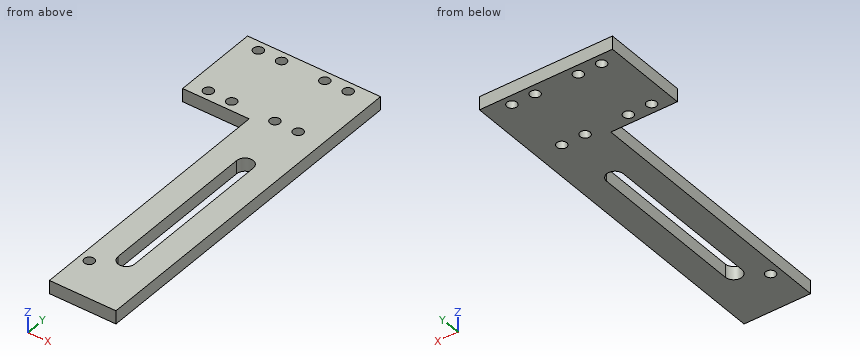
Autodesk Inventor part; units mm, degrees
ref_plane "YZ Plane" through (0, 0, 0) normal (1, 0, 0) x (0, 1, 0)
ref_plane "XZ Plane" through (0, 0, 0) normal (0, 1, 0) x (-1, 0, 0)
ref_plane "XY Plane" through (0, 0, 0) normal (0, 0, 1) x (1, 0, 0)
sketch "Skizze1" plane through (0, 0, 0) normal (0, 0, 1) x (1, 0, 0)
  line L0 (0, 0) -> (0, 80)
  line L1 (0, 80) -> (-20, 80)
  line L2 (-20, 80) -> (-20, 106)
  line L3 (-20, 106) -> (20, 106)
  line L4 (20, 106) -> (20, 0)
  line L5 (20, 0) -> (0, 0)
  arc A0 (7.5, 17.5) -> (12.5, 17.5) centre (10, 17.5) ccw
  arc A1 (12.5, 65) -> (7.5, 65) centre (10, 65) ccw
  line L6 (7.5, 65) -> (7.5, 17.5)
  line L7 (12.5, 65) -> (12.5, 17.5)
  dimension "d0" = 26
  dimension "d1" = 80
  dimension "d2" = 40
  dimension "d3" = 20
  dimension "d5" = 5
  dimension "d6" = 15
  dimension "d7" = 10
  dimension "d8" = 10
  dimension "d9" = 65
  dimension "d12" = 2.5
extrude "Extrusion1" add sketch "Skizze1" along normal blind 4
hole "Bohrung1" at (-14.5, 83, 4) direction (0, 0, -1) diameter 3 depth 8 tip angle 118
hole "Bohrung2" at (-7.5, 83, 4) direction (0, 0, -1) diameter 3 depth 8 tip angle 118
hole "Bohrung3" at (5.5, 83, 4) direction (0, 0, -1) diameter 3 depth 8 tip angle 118
hole "Bohrung4" at (12.5, 83, 4) direction (0, 0, -1) diameter 3 depth 8 tip angle 118
hole "Bohrung5" at (-14.5, 103, 4) direction (0, 0, -1) diameter 3 depth 8 tip angle 118
hole "Bohrung6" at (-7.5, 103, 4) direction (0, 0, -1) diameter 3 depth 8 tip angle 118
hole "Bohrung7" at (5.5, 103, 4) direction (0, 0, -1) diameter 3 depth 8 tip angle 118
hole "Bohrung8" at (12.5, 103, 4) direction (0, 0, -1) diameter 3 depth 8 tip angle 118
hole "Bohrung9" at (3, 12, 4) direction (0, 0, -1) diameter 3 depth 8 tip angle 118
properties part number "Montageplatte"
The model under review builds one solid part; all positions refer to its coordinate system, in mm. Round coordinates to 2 decimals unless told otherwise and drop trailing zeros. Loops run counter-clockwise (first coordinate to the right, second up) from the corner with the lowest first, then second, coordinate; pieces in that order, holes last. Notation, with made-up numbers: (84.5, -32.75) - (135.5, -32.75) arc R29 ccw to (135.5, -4.75) - close; hole circle Ø9 at (50, -34). An arc over 180 degrees is marked (long way). Use a Markdown table: item, result. Add a question column.
Q1. Add section A-A (x = 3). State the section outline as (y, z) points, plus the area to 3 significant figures.
Q2. For probe 1 along X at (y, z) = (83, 2.35); probe 2 along Y at (x, z) = (-14.5, 1.5); probe 3 along X at (y, z) = (63.5, 3.85), list the stretches that pass through material, from the lowest coordinate up.
Q3. Insertion check: pin 1 Ø4 at (x, y) = (3, 12) entering from +Z; pin 2 Ø1.2 at (y, z) = (29.5, 2) entering from -X. Each pin has a flat end and moves straight along its axis. Give the tip position at first contact, or say it passes through.
Q4. Add section B-B (y = 24). State the section outline as (x, z) points, plus the area to 3 significant figures.
Q5. Add section C-C (y = 83). State the section outline as (x, z) points, plus the area to 3 significant figures.
Q6. Add section D-D (z = 0.6). State how many separate pieces and enclosed holes the cut face has, plus the area to 3 significant figures.
Worked answers:
| question | item | result |
|---|---|---|
| 1 | outline | (0, 0) - (10.5, 0) - (10.5, 4) - (0, 4) - close; (13.5, 0) - (106, 0) - (106, 4) - (13.5, 4) - close |
| 1 | area | 412 mm² |
| 2 | probe 1 | -20 to -16, -13 to -9, -6 to 4, 7 to 11, 14 to 20 |
| 2 | probe 2 | 80 to 81.5, 84.5 to 101.5, 104.5 to 106 |
| 2 | probe 3 | 0 to 7.5, 12.5 to 20 |
| 3 | pin 1 | z = 4 |
| 3 | pin 2 | x = 0 |
| 4 | outline | (0, 0) - (7.5, 0) - (7.5, 4) - (0, 4) - close; (12.5, 0) - (20, 0) - (20, 4) - (12.5, 4) - close |
| 4 | area | 60.0 mm² |
| 5 | outline | (-20, 0) - (-16, 0) - (-16, 4) - (-20, 4) - close; (-13, 0) - (-9, 0) - (-9, 4) - (-13, 4) - close; (-6, 0) - (4, 0) - (4, 4) - (-6, 4) - close; (7, 0) - (11, 0) - (11, 4) - (7, 4) - close; (14, 0) - (20, 0) - (20, 4) - (14, 4) - close |
| 5 | area | 112 mm² |
| 6 | separate pieces | 1 |
| 6 | enclosed holes | 10 |
| 6 | area | 2,320 mm² |
